Read the model definition and answer for the solid it produces. Units are mm, in the model's axes. Face numbers are marked on the shaded views. A direction names the side the tool comes from. Coordinates: 2 decimals unless noted, no trailing zeros. Order: outer loops, then holes, each group sorted by start corner. A loop starts at its lowest first (then second) coordinate and runs counter-clockwise, first axis right, second up. Notation, with made-up numbers: (-1.75, -22.5) - (32.25, -22.5) arc R14 ccw to (32.25, -1.5) - close; hole circle Ø5 at (76.25, 46.5). An arc over 180 degrees is marked (long way). Use one line per item in the form item = value.
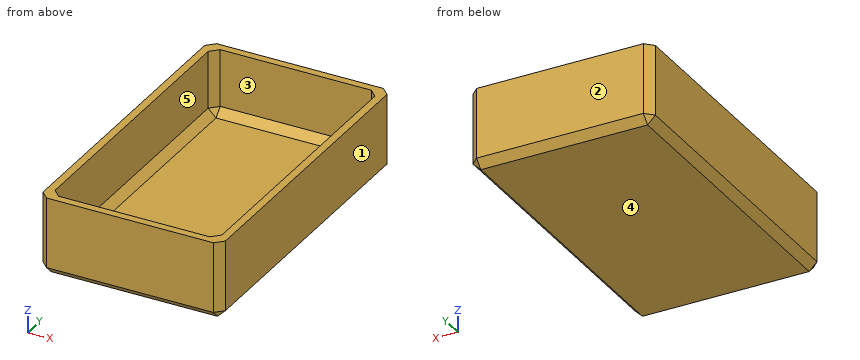
Autodesk Fusion 360 part; units mm, degrees
sketch "Sketch1" plane through (0, 0, 0) normal (0, 0, 1) x (1, 0, 0)
  line L0 (35, 60) -> (-35, 60)
  line L1 (-35, 60) -> (-35, -60)
  line L2 (-35, -60) -> (35, -60)
  line L3 (35, -60) -> (35, 60)
  line L4 (35, 60) -> (-35, -60) construction
  line L5 (-35, 60) -> (35, -60) construction
  dimension "d1" = 70
  dimension "d2" = 120
extrude "Extrude1" add sketch "Sketch1" along normal blind 5
sketch "Sketch2" plane through (0, 0, 5) normal (0, 0, 1) x (-1, 0, 0)
  line L0 (-35, 60) -> (-35, -60)
  line L1 (-35, -60) -> (35, -60)
  line L2 (35, -60) -> (35, 60)
  line L3 (35, 60) -> (-35, 60)
  line L4 (32, 57) -> (-32, 57)
  line L5 (-32, 57) -> (-32, -57)
  line L6 (-32, -57) -> (32, -57)
  line L7 (32, -57) -> (32, 57)
  dimension "d5" = -3
extrude "Extrude2" add sketch "Sketch2" along normal blind 25
chamfer "Chamfer1" distance 3 angle 45 12 edges at (35, -60, 15) (-35, -60, 15) (35, 60, 15) (-35, 60, 15) (-32, 57, 17.5) (0, 57, 5) (-32, 0, 5) (32, 57, 17.5) (32, 0, 5) (32, -57, 17.5) (0, -57, 5) (-32, -57, 17.5) 1 faces at (-11.6667, -20, 0)
(1) Section A-A, the plane z = 10.75 is taken. Write down the section's boundary in (x, y).
Answer list:
outline = (-35, -57) - (-32, -60) - (32, -60) - (35, -57) - (35, 57) - (32, 60) - (-32, 60) - (-35, 57) - close; hole (-32, -54) - (-29, -57) - (29, -57) - (32, -54) - (32, 54) - (29, 57) - (-29, 57) - (-32, 54) - close
(2) Given pin 1 Ø4 at (x, y) = (11, 6.5) entering from -Z; pin 2 Ø4 at (x, y) = (-20.5, -22.5) entering from +Z, each flat-ended and moving along its own axis, determine where each tip first touches the part or whether it passes through.
Answer list:
pin_1 = 0
pin_2 = 5
(3) The mould has two halves that part along X. Classify the marked faces 1, 2 and 3: +X half, -X half, draft (parallel to the pull), parting line (faces both ways), or undercut.
Answer list:
face_1 = +X half
face_2 = draft
face_3 = undercut
(4) Straight lines are drawn through the part: L1, parallel to Y at x = -3, z = 22; L2, parallel to X at y = 53, z = 28.5; L3, parallel to Z at x = 4, y = -32. For each, find the intervals that lie inside material, in ascending order.
Answer list:
L1 = -60 to -57, 57 to 60
L2 = -35 to -32, 32 to 35
L3 = 0 to 5
(5) Section C-C, the plane x = -26.5 is taken. Write down the section's boundary in (y, z), then the cut area to 3 significant figures.
Answer list:
outline = (-60, 3) - (-57, 0) - (57, 0) - (60, 3) - (60, 30) - (57, 30) - (57, 8) - (54, 5) - (-54, 5) - (-57, 8) - (-57, 30) - (-60, 30) - close
area = 750 mm2
(6) Section B-B, the plane y = 23 is taken. Write down the section's boundary in (x, z).
Answer list:
outline = (-35, 3) - (-32, 0) - (32, 0) - (35, 3) - (35, 30) - (32, 30) - (32, 8) - (29, 5) - (-29, 5) - (-32, 8) - (-32, 30) - (-35, 30) - close
(7) Which of the six approach directions +Z, -Z, +X, -X, +Y, -Y give full straight-line access (tool end or side, diameter ignored) to the marked faces 4 and 5?
Answer list:
face_4 = -Z, +X, -X, +Y, -Y
face_5 = +Z
